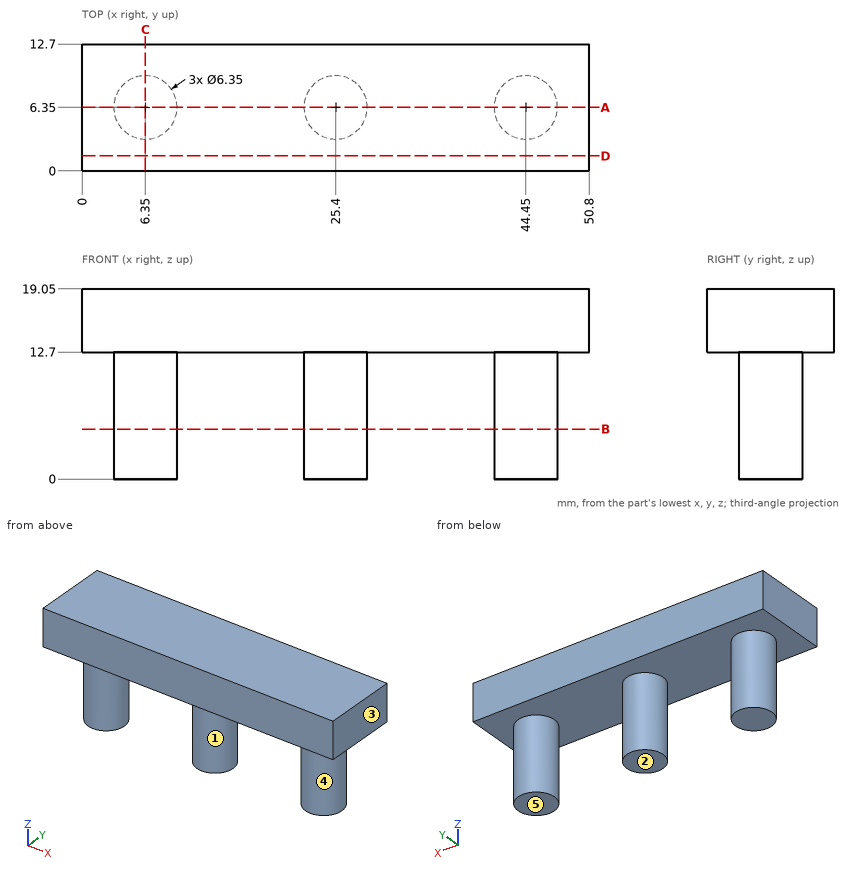
Geometry check sheet. Reference: drawing and pictorial views, mm from the part's lowest x, y, z. A direction names the side the tool comes from. Round coordinates to 2 decimals unless told otherwise and drop trailing zeros. Order: outer loops, then holes, each group sorted by start corner. A loop starts at its lowest first (then second) coordinate and runs counter-clockwise, first axis right, second up. Notation, with made-up numbers: (43.25, 14) - (61.25, 14) arc R21 cw to (61.25, 22) - close; hole circle Ø10 at (43.5, 23). An arc over 180 degrees is marked (long way). Write item = value, one per line.
Q1. Section check C-C (x = 6.35). Record the boundary of the cut face in (y, z) (3 decimals), and give its area (3 significant figures).
Computed:
outline = (0, 12.7) - (3.175, 12.7) - (3.175, 0) - (9.525, 0) - (9.525, 12.7) - (12.7, 12.7) - (12.7, 19.05) - (0, 19.05) - close
area = 161 mm^2
Q2. Draft check along X on the marked faces 1, 2 and 3. Enter one of: pulls with the +X half, pulls with the -X half, needs draft (parallel to the pull), parting line crosses it, or undercut.
Computed:
face_1 = undercut
face_2 = needs draft
face_3 = pulls with the +X half
Q3. Section check B-B (z = 5). Record the boundary of the cut face in (x, y) (3 decimals).
Computed:
outline = circle Ø6.35 at (6.35, 6.35); circle Ø6.35 at (25.4, 6.35); circle Ø6.35 at (44.45, 6.35)
Q4. Section check D-D (y = 1.5). Record the boundary of the cut face in (x, z).
Computed:
outline = (0, 12.7) - (50.8, 12.7) - (50.8, 19.05) - (0, 19.05) - close
Q5. Tool access check on the marked faces 4 and 5. Record the directions out of +Z, -Z, +X, -X, +Y, -Y that give a thin tool (end or side, any length) a straight path to the whole face; none if there is none.
Computed:
face_4 = -Z
face_5 = -Z, +X, -X, +Y, -Y
Q6. Go/stop test with flat-tipped pins: pin 1 (1 mm diameter, centred on x = 13.5, z = 10.5, fed in from +Y); pin 2 (2 mm diameter, centred on y = 5.5, z = 7.5, fed in from +X) (3 decimals); pin 3 (1.5 mm diameter, centred on x = 6.5, z = 3, fed in from +Y) (3 decimals); pin 4 (2 mm diameter, centred on x = 17, y = 8, fed in from -Z). Record where each tip stops, or that it passes through.
Computed:
pin_1 = through
pin_2 = 47.625
pin_3 = 9.525
pin_4 = 12.7
Q7. Thickness scan on line 1 along X through (y, z) = (6.25, 7.5); line 2 along X through (y, z) = (5, 1.25); line 3 along Z through (x, y) = (38, 10.75). Record the ranges inside material, lowest first.
Computed:
line_1 = 3.18 to 9.52, 22.23 to 28.57, 41.28 to 47.62
line_2 = 3.48 to 9.22, 22.53 to 28.27, 41.58 to 47.32
line_3 = 12.7 to 19.05
Q8. Section check A-A (y = 6.35). Record the boundary of the cut face in (x, z) (3 decimals), and give its area (3 significant figures).
Computed:
outline = (0, 12.7) - (3.175, 12.7) - (3.175, 0) - (9.525, 0) - (9.525, 12.7) - (22.225, 12.7) - (22.225, 0) - (28.575, 0) - (28.575, 12.7) - (41.275, 12.7) - (41.275, 0) - (47.625, 0) - (47.625, 12.7) - (50.8, 12.7) - (50.8, 19.05) - (0, 19.05) - close
area = 565 mm^2
